Autodesk Inventor part; units mm, degrees
ref_plane "YZ Plane" through (0, 0, 0) normal (1, 0, 0) x (0, 1, 0)
ref_plane "XZ Plane" through (0, 0, 0) normal (0, 1, 0) x (-1, 0, 0)
ref_plane "XY Plane" through (0, 0, 0) normal (0, 0, 1) x (1, 0, 0)
sketch "Sketch1" plane through (0, 0, 0) normal (0, 1, 0) x (-1, 0, 0)
  line L0 (0, 0) -> (38.2, 0)
  line L1 (38.2, 0) -> (38.2, -25.2)
  line L2 (38.2, -25.2) -> (0, -25.2)
  line L3 (0, -25.2) -> (0, 0)
  circle A0 centre (33.1, -20.1) radius 1.3
  circle A1 centre (5.1, -5.1) radius 1.3
  circle A2 centre (5.1, -20.1) radius 1.3
  line L4 (0, 0) -> (38.2, -25.2) construction
  line L5 (38.2, 0) -> (0, -25.2) construction
  line L6 (5.1, -5.1) -> (33.1, -20.1) construction
  point P0 (19.1, -12.6)
  dimension "d1" = 15
  dimension "d2" = 28
  dimension "d3" = 2.6
  dimension "d4" = 2.6
  dimension "d5" = 2.6
  dimension "d18" = 25.2
  dimension "d19" = 38.2
extrude "Extrusion1" add sketch "Sketch1" along normal blind 3
sketch "Sketch2" plane through (0, 3, 0) normal (0, 1, 0) x (1, 0, 0)
  circle A0 centre (-5.1, 5.1) radius 1.3
  circle A1 centre (-5.1, 5.1) radius 3
  circle A2 centre (-5.1, 20.1) radius 1.3
  circle A3 centre (-5.1, 20.1) radius 3
  circle A4 centre (-33.1, 20.1) radius 1.3
  circle A5 centre (-33.1, 20.1) radius 3
  point P0 (0, 0)
  dimension "d12" = 6
  dimension "d13" = 6
  dimension "d14" = 6
extrude "Extrusion2" add sketch "Sketch2" along normal blind 4
pattern_linear "Rectangular Pattern1" count 2 spacing 25.2 along (0, 0, 1) of "Extrusion1", "Extrusion2"
fillet "Fillet2" radius 2 4 edges at (0, 1.5, 25.2) (0, 1.5, -25.2) (-38.2, 1.5, -25.2) (-38.2, 1.5, 25.2)
equation "\"d4\" = d3"
equation "\"d5\" = d3"
equation "\"d13\" = d12"
equation "\"d14\" = d12"
equation "\"d7\" = d8"
properties part number "adc_board_rack"
Check sheet for the modelled part. Datum: model origin and axes. Units: mm. A direction names the side the tool comes from. Coordinates: 2 decimals unless noted, no trailing zeros. Loops run counter-clockwise (first coordinate to the right, second up) from the corner with the lowest first, then second, coordinate; pieces in that order, holes last.
1) Material ranges on probe 1 along X at (y, z) = (3.25, -20.1); probe 2 along Z at (x, y) = (-5.1, 2.5); probe 3 along X at (y, z) = (2.75, -20.1), recorded low to high.
2) Sectioned sample at A-A (y = 6.25). Count the separate pieces of the cut face and the enclosed holes in it, and give its area (3 significant figures).
3) Sectioned sample at B-B (y = 1.25). Record the boundary of the cut face in (x, z).
4) Release check for a two-part mould opening along X. For faces 1 (the face through (-5.014, 3.451, -3.803)), 2 (the face through (0, 1, 0)), 3 (the face through (-4, 7, -19)) record: released by +X, released by -X, zero draft, split by the parting line, or undercut.
5) Gauge pin test, flat ends, axial feed: pin 1 (3 mm diameter, centred on x = -7.5, z = -11.5, fed in from -Y); pin 2 (2.5 mm diameter, centred on x = -5.1, z = -20.1, fed in from -Y); pin 3 (10 mm diameter, centred on x = -30.5, z = -12, fed in from +Y). Record the tip position at first contact, or that the pin passes through.
6) Sectioned sample at D-D (z = -0.5). Record the boundary of the cut face in (x, y), and give its area (3 significant figures).
7) Access from +Z, -Z, +X, -X, +Y, -Y to the whole of each face (thin tool, end or side, straight path). Record for faces 4 (the face through (-37.6, 1.52, -24.63)), 5 (the face through (-5.75, 4.97, -23.03)).
Check sheet entries:
1. probe 1: x = -36.1 to -34.4, -31.8 to -30.1, -8.1 to -6.4, -3.8 to -2.1
1. probe 2: z = -25.2 to -21.4, -18.8 to -6.4, -3.8 to 3.8, 6.4 to 18.8, 21.4 to 25.2
1. probe 3: x = -38.2 to -34.4, -31.8 to -6.4, -3.8 to 0
2. separate pieces: 6
2. enclosed holes: 6
2. area: 138 mm2
3. outline: (-38.2, -23.2) arc R2 ccw to (-36.2, -25.2) - (-2, -25.2) arc R2 ccw to (0, -23.2) - (0, 23.2) arc R2 ccw to (-2, 25.2) - (-36.2, 25.2) arc R2 ccw to (-38.2, 23.2) - close; hole circle Ø2.6 at (-33.1, -20.1); hole circle Ø2.6 at (-33.1, 5.1); hole circle Ø2.6 at (-5.1, -20.1); hole circle Ø2.6 at (-5.1, -5.1); hole circle Ø2.6 at (-5.1, 5.1); hole circle Ø2.6 at (-5.1, 20.1)
4. face 1: undercut
4. face 2: released by +X
4. face 3: zero draft
5. pin 1: stops at y = 0
5. pin 2: passes through
5. pin 3: stops at y = 3
6. outline: (-38.2, 0) - (0, 0) - (0, 3) - (-38.2, 3) - close
6. area: 115 mm2
7. face 4: -Z, -X, +Y, -Y
7. face 5: +Y
